CAD build for the part. Positions are in the model's coordinates, mm. A direction names the side the tool comes from. Coordinates: 2 decimals unless noted, no trailing zeros. Loops run counter-clockwise (first coordinate to the right, second up) from the corner with the lowest first, then second, coordinate; pieces in that order, holes last. Notation, with made-up numbers: (15.5, 43.5) -> (71.5, 43.5) arc R27 cw to (71.5, 76.5) -> close; hole circle Ø11 at (18, 46.5). An arc over 180 degrees is marked (long way). Return JSON: item names as keys, results as strings. Group by question number.
(1) Saw through at B-B on y = -1.2. Write the cut outline in (x, z).
(2) Probe L1, parallel to X at y = 1.8, z = 0.8; L2, parallel to Z at x = 6.75, y = -0.1; L3, parallel to Z at x = 8.5, y = 0.5. List the from-to ranges inside material, lowest first.
(3) Saw through at A-A on z = -0.35. Write the cut outline in (x, y).
(4) Mould opens along X. For faces 1 (the face through (25, 0, 0)), 2 (the face through (2.746, -0.571, 1.812)), 3 (the face through (12, 2, 0)), 4 (the face through (0, 0, 0)) say: pulls with the +X half, pulls with the -X half, needs draft (parallel to the pull), parting line crosses it, or undercut.
(5) Saw through at C-C on x = 12. Write the cut outline in (y, z), then the cut area to 3 significant figures.
(6) Tool access for faces 5 (the face through (24, 2, 0)), 6 (the face through (22.246, -0.571, 1.812)): list every direction of +Z, -Z, +X, -X, +Y, -Y with a clear straight run to the whole face (end or side of a thin tool).
```python
from build123d import *


with BuildPart() as part:
    # Çizim1 → Döndür1 (revolve)
    with BuildSketch(Plane.XY, mode=Mode.PRIVATE) as d_nd_r1_sk:
        Polygon((0, 0), (25, 0), (25, 2), (22.5, 2), (22.5, 1.9), (22, 1.9), (22, 2), (3, 2), (3, 1.9), (2.5, 1.9), (2.5, 2), (0, 2), align=None)
    revolve(d_nd_r1_sk.sketch.rotate(Axis((0, 0, 0), (1, 0, 0)), 90), axis=Axis((0, 0, 0), (1, 0, 0)))


solid = part.part
```
Geometry results:
{
 "1": {"outline": "(0, -1.6) -> (2.5, -1.6) -> (2.5, -1.47) -> (3, -1.47) -> (3, -1.6) -> (22, -1.6) -> (22, -1.47) -> (22.5, -1.47) -> (22.5, -1.6) -> (25, -1.6) -> (25, 1.6) -> (22.5, 1.6) -> (22.5, 1.47) -> (22, 1.47) -> (22, 1.6) -> (3, 1.6) -> (3, 1.47) -> (2.5, 1.47) -> (2.5, 1.6) -> (0, 1.6) -> close"},
 "2": {"L1": "0 to 2.5, 3 to 22, 22.5 to 25", "L2": "-2 to 2", "L3": "-1.94 to 1.94"},
 "3": {"outline": "(0, -1.97) -> (2.5, -1.97) -> (2.5, -1.87) -> (3, -1.87) -> (3, -1.97) -> (22, -1.97) -> (22, -1.87) -> (22.5, -1.87) -> (22.5, -1.97) -> (25, -1.97) -> (25, 1.97) -> (22.5, 1.97) -> (22.5, 1.87) -> (22, 1.87) -> (22, 1.97) -> (3, 1.97) -> (3, 1.87) -> (2.5, 1.87) -> (2.5, 1.97) -> (0, 1.97) -> close"},
 "4": {"face 1": "pulls with the +X half", "face 2": "undercut", "face 3": "needs draft", "face 4": "pulls with the -X half"},
 "5": {"outline": "circle Ø4 at (0, 0)", "area": "12.6 mm²"},
 "6": {"face 5": "+X, -X", "face 6": "none"}
}
